Geometry: final body of the model. Coordinates: model frame, mm. A direction names the side the tool comes from. Give positions to 0.01 mm unless a question says otherwise; leave off trailing zeros. Write each loop counter-clockwise with the first axis right and the second up, starting at its lowest first coordinate (ties: lowest second). Pieces come first, ordered by that corner, then holes. Notation, with made-up numbers: (24, 3.25) - (44, 3.25) arc R28 ccw to (44, 37.25) - close; hole circle Ø3 at (-5.75, 73.5). An arc over 180 degrees is marked (long way). Return JSON: item names as keys, results as strings.
from build123d import *

# Parameters (mm, degrees)
PAD005_DEPTH    = 12
SKETCH025_R     = 2.5
POCKET019_DEPTH = 10
POCKET020_DEPTH = 1
SKETCH027_W     = 8
SKETCH027_H     = 8.3
POCKET021_DEPTH = 5
PAD006_DEPTH    = 2.5
SKETCH029_W     = 12.5
SKETCH029_H     = 5
POCKET022_DEPTH = 2


with BuildPart() as part:
    # Sketch024 → Pad005 (new body)
    with BuildSketch(Plane.XY):
        with BuildLine():
            ThreePointArc((0, 0), (0.0125001507, 3.6000868045), (0.05, 7.2))
            Line((0.05, 7.2), (0.75, 22.55))
            add(Edge.make_bspline(
                [(0.75, 22.55), (0.790433, 24.50555), (2.8995135699, 28.3383927733), (10.6468681476, 35.231617337), (14.5053016695, 34.8194742751), (20.1, 35.5)],
                knots=[0, 0, 0, 0, 0.3333333333, 0.6666666667, 1, 1, 1, 1], degree=3))
            Line((20.1, 35.5), (64.2, 35.5))
            add(Edge.make_bspline(
                [(92, 0), (92.391037, 11.810127), (88.126587, 35.076866), (64.2, 35.5)],
                knots=[0, 0, 0, 0, 1, 1, 1, 1], degree=3))
            Line((92, 0), (0, 0))
        make_face()
    extrude(amount=PAD005_DEPTH)

    # Sketch025 (on Face8 of Pad005) → Pocket019 (cut)
    with BuildSketch(Plane.XY.offset(12)):
        with Locations((17, 25)):
            Circle(SKETCH025_R)
        with BuildLine():
            ThreePointArc((84.5, 0), (82, 2.5), (79.5, 0))
            Line((79.5, 0), (84.5, 0))
        make_face()
        with BuildLine():
            Line((2, 0), (2.5758571429, 18.6857169977))
            ThreePointArc((7.6817324497, 29.5040514173), (4.0036624605, 24.625907301), (2.5758571429, 18.6857169977))
            ThreePointArc((11, 28), (9.8256709089, 29.8216112511), (7.6817324497, 29.5040514173))
            Line((11, 25), (11, 28))
            ThreePointArc((11, 25), (17, 19), (23, 25))
            Line((23, 25), (23, 31.5))
            ThreePointArc((25, 33.5), (23.5857864376, 32.9142135624), (23, 31.5))
            Line((25.1, 33.5), (25, 33.5))
            ThreePointArc((27.1, 31.5), (26.5142135624, 32.9142135624), (25.1, 33.5))
            Line((27.1, 12), (27.1, 31.5))
            ThreePointArc((27.1, 12), (27.6857864376, 10.5857864376), (29.1, 10))
            Line((31.1, 10), (29.1, 10))
            ThreePointArc((31.1, 10), (32.5142135624, 10.5857864376), (33.1, 12))
            Line((33.1, 31.5), (33.1, 12))
            ThreePointArc((35.1, 33.5), (33.6857864376, 32.9142135624), (33.1, 31.5))
            Line((49.3, 33.5), (35.1, 33.5))
            ThreePointArc((51.3, 31.5), (50.7142135624, 32.9142135624), (49.3, 33.5))
            Line((51.3, 12), (51.3, 31.5))
            ThreePointArc((51.3, 12), (51.8857864376, 10.5857864376), (53.3, 10))
            Line((55.3, 10), (53.3, 10))
            ThreePointArc((55.3, 10), (56.7142135624, 10.5857864376), (57.3, 12))
            Line((57.3, 31.4999999999), (57.3, 12))
            ThreePointArc((59.3, 33.4999999999), (57.8857864376, 32.9142135623), (57.3, 31.4999999999))
            Line((59.3, 33.5), (64.2, 33.5))
            ThreePointArc((87.491325765, 7.8139309331), (81.5019467421, 25.7859071373), (64.2, 33.5))
            ThreePointArc((85.5, 6), (86.8468225322, 6.521463877), (87.491325765, 7.8139309331))
            Line((82, 6), (85.5, 6))
            ThreePointArc((82, 6), (77.7573593129, 4.2426406871), (76, 0))
            Line((22, 0), (76, 0))
            Line((22, 1), (22, 0))
            Line((16, 1), (22, 1))
            Line((16, 0), (16, 1))
            Line((2, 0), (16, 0))
        make_face()
    extrude(amount=-POCKET019_DEPTH, mode=Mode.SUBTRACT)

    # Sketch026 (on Face3 of Pocket019) → Pocket020 (cut)
    with BuildSketch(Plane.XZ):
        Polygon((22, 12), (22, 4), (18, 10), (16, 10), (16, 12), align=None)
    extrude(amount=-POCKET020_DEPTH, mode=Mode.SUBTRACT)

    # Sketch027 → Pocket021 (cut)
    with BuildSketch(Plane.YZ):
        with Locations((4, 6.15)):
            Rectangle(SKETCH027_W, SKETCH027_H)
    extrude(amount=POCKET021_DEPTH, mode=Mode.SUBTRACT)

    # Sketch028 (on Face8 of Pocket021) → Pad006 (join)
    with BuildSketch(Plane.XY.offset(12)):
        with BuildLine():
            ThreePointArc((31.1, 10), (32.5142135624, 10.5857864376), (33.1, 12))
            Line((33.1, 12), (33.1, 14))
            ThreePointArc((33.1, 14), (32.5142135624, 15.4142135624), (31.1, 16))
            Line((29.1, 16), (31.1, 16))
            ThreePointArc((29.1, 16), (27.6857864376, 15.4142135624), (27.1, 14))
            Line((27.1, 12), (27.1, 14))
            ThreePointArc((27.1, 12), (27.6857864376, 10.5857864376), (29.1, 10))
            Line((29.1, 10), (31.1, 10))
        make_face()
        with BuildLine():
            ThreePointArc((51.3, 12), (51.8857864376, 10.5857864376), (53.3, 10))
            Line((53.3, 10), (55.3, 10))
            ThreePointArc((55.3, 10), (56.7142135624, 10.5857864376), (57.3, 12))
            Line((57.3, 12), (57.3, 14))
            ThreePointArc((57.3, 14), (56.7142135624, 15.4142135624), (55.3, 16))
            Line((53.3, 16), (55.3, 16))
            ThreePointArc((53.3, 16), (51.8857864376, 15.4142135624), (51.3, 14))
            Line((51.3, 12), (51.3, 14))
        make_face()
    extrude(amount=PAD006_DEPTH)

    # Mirrored002: part across XZ


with BuildPart() as part_1:
    add(part.part)
    add(part.part.mirror(Plane.XZ))

    # Sketch029 (on Face33 of Mirrored002) → Pocket022 (cut)
    with BuildSketch(Plane(origin=(0, 35.5, 0), x_dir=(-1, 0, 0), z_dir=(0, 1, 0))):
        with Locations((-42.65, 7)):
            Rectangle(SKETCH029_W, SKETCH029_H)
    extrude(amount=-POCKET022_DEPTH, mode=Mode.SUBTRACT)


with BuildPart() as part_2:
    # Body004 placement: moved
    add(part_1.part.moved(Location((0, 0, -12))))


solid = part_2.part
Q1. Material intervals for probe 1 along Y at (x, z) = (17, -4); probe 2 along X at (y, z) = (-25, -2.25); probe 3 along Y at (x, z) = (64, -2.75), sorted ascending. Write a range as [from, to].
Answer key:
{"probe 1": "y = [-35.17, -27.5], [-22.5, -19], [-1, 1], [19, 22.5], [27.5, 35.17]", "probe 2": "x = [1.31, 4.19], [11, 14.5], [19.5, 23], [27.1, 33.1], [51.3, 57.3], [82.18, 85.36]", "probe 3": "y = [-35.5, -33.5], [33.5, 35.5]"}
Q2. Pin query (flat end, axial travel): P1, Ø8, axis at y = 12.5, z = -4, coming from the +X side; P2, Ø3, axis at y = 3, z = 1, coming from the +X side; P3, Ø1, axis at y = 26, z = -7.5, coming from the +X side. Return the tip coordinate at first contact, or that it passes through.
Answer key:
{"P1": "stops at x = 91.51", "P2": "stops at x = 92.02", "P3": "stops at x = 84.99"}
Q3. Section query A-A, the plane x = 47. Return the cut outline in (y, z).
Answer key:
{"outline": "(-35.5, -12) - (35.5, -12) - (35.5, -7.5) - (33.5, -7.5) - (33.5, -10) - (-33.5, -10) - (-33.5, 0) - (-35.5, 0) - close; (33.5, -2.5) - (35.5, -2.5) - (35.5, 0) - (33.5, 0) - close"}
Q4. Mould query, pull axis Y, two halves, no side actions, for faces 5 (the flat face through (0.395, -14.768, -6.084)), 6 (the cylindrical face through (23.6, 32.93, -4.93)), 7 (the cylindrical face through (56.73, 15.4, 1.23)). Classes: pulls with the +Y half, pulls with the -Y half, needs draft (parallel to the pull), parting line crosses it, or undercut.
Answer key:
{"face 5": "pulls with the -Y half", "face 6": "undercut", "face 7": "pulls with the +Y half"}
Q5. Set-up query: faces 1 (the cylindrical face through (56.73, -15.4, 1.23)), 2 (the cylindrical face through (32.53, 15.4, 1.23)), 3 (the flat face through (47, 0, -12)), 4 (the flat face through (42, -33.5, -5)). Return all of +Z, -Z, +X, -X, +Y, -Y with unobstructed straight access to the full face (end or side cutting, diameter ignored); none if empty.
Answer key:
{"face 1": "+Z, +X, -Y", "face 2": "+Z, +Y", "face 3": "-Z, +X, -X, +Y, -Y", "face 4": "+Z"}
Q6. Section query B-B, the plane z = -9. Count the separate pieces of the cut face and the enclosed holes in it, plus the area to 3 significant figures.
Answer key:
{"separate pieces": "2", "enclosed holes": "3", "area": "1,580 mm^2"}
